Read the model definition and answer for the solid it produces. Units are mm, in the model's axes. Coordinates: 2 decimals unless noted, no trailing zeros. Loops run counter-clockwise (first coordinate to the right, second up) from the corner with the lowest first, then second, coordinate; pieces in that order, holes last.
Q1. Straight lines are drawn through the part: line 1 (Y direction, x = -27, z = 1.6); line 2 (X direction, y = 35.5, z = 1.4); line 3 (X direction, y = 50, z = 0.25). For each, find the intervals that lie inside material, in ascending order.
Q2. Section A-A (y = 59.5) is taken. Give the vertices of the cut face in (x, z).
Q3. Flat-ended cylindrical pins translate along their axes: P1, Ø2, axis at x = -15, y = 26.5, coming from the -Z side; P2, Ø0.6, axis at x = -27, z = 1.5, coming from the -Y side; P3, Ø0.6, axis at x = -35, z = 0.5, coming from the -Y side. Find the tip coordinate at first contact, or state that the pin passes through.
Q4. Section C-C (z = 0.65) is taken. Count the separate pieces of the cut face and the enclosed holes in it, then the cut area to 3 significant figures.
Q5. Section B-B (x = -42) is taken. Give the vertices of the cut face in (y, z), then the cut area to 3 significant figures.
from build123d import *

# Parameters (mm, degrees)
F0_R     = 1.6
F0_W     = 2
F0_H     = 3
F1_DEPTH = 2
F2_R     = 5
F3_R     = 2
F4_R     = 13.153232


with BuildPart() as f1:
    # F0 (on Top) → F1 (new body)
    with BuildSketch(Plane.XY):
        with Locations((-42.057751, 35.748998)):
            Circle(F0_R)
        with BuildLine():
            ThreePointArc((-13.157751, 35.748998), (-11.557751, 34.148998), (-9.957751, 35.748998))
            ThreePointArc((-9.957751, 35.748998), (-11.557751, 37.348998), (-13.157751, 35.748998))
        make_face()
        with Locations((-42.057751, 5.248998)):
            Circle(F0_R)
        with BuildLine():
            ThreePointArc((-13.157751, 5.248998), (-11.557751, 3.648998), (-9.957751, 5.248998))
            ThreePointArc((-9.957751, 5.248998), (-11.557751, 6.848998), (-13.157751, 5.248998))
        make_face()
        with BuildLine():
            ThreePointArc((-45.849798, 66.493904), (-45.855762, 66.371516), (-45.857751, 66.248998))
            Line((-45.857751, 66.248998), (-45.857751, 60.434222))
            Line((-45.857751, 60.434222), (-45.857751, 35.748998))
            Line((-45.857751, 35.748998), (-45.857751, 33.160256))
            Line((-45.857751, 33.160256), (-45.857751, 5.248998))
            Line((-45.857751, 5.248998), (-45.857751, -19.436226))
            Line((-45.857751, -19.436226), (-45.857751, -25.251002))
            Line((-45.857751, -25.251002), (-45.857751, -26.920806))
            ThreePointArc((-45.857751, -26.920806), (-40.539361, -28.348832), (-35.116938, -29.308968))
            ThreePointArc((-35.116938, -29.308968), (-26.575174, -26.898307), (-18.01507, -29.243015))
            ThreePointArc((-18.01507, -29.243015), (-12.838073, -28.295417), (-7.757751, -26.920806))
            Line((-7.757751, -26.920806), (-7.757751, -25.251002))
            Line((-7.757751, -25.251002), (-7.757751, -19.436226))
            Line((-7.757751, -19.436226), (-7.757751, 5.248998))
            Line((-7.757751, 5.248998), (-7.757751, 35.748998))
            Line((-7.757751, 35.748998), (-7.757751, 60.434222))
            Line((-7.757751, 60.434222), (-7.757751, 66.248998))
            ThreePointArc((-7.757751, 66.248998), (-7.759739, 66.371516), (-7.765703, 66.493904))
            ThreePointArc((-7.765703, 66.493904), (-11.655268, 70.022009), (-15.307751, 66.248998))
            ThreePointArc((-15.307751, 66.248998), (-26.807751, 65.147515), (-38.307751, 66.248998))
            ThreePointArc((-38.307751, 66.248998), (-41.960233, 70.022009), (-45.849798, 66.493904))
        make_face()
        with Locations((-42.057751, -23.592251)):
            Circle(F0_R, mode=Mode.SUBTRACT)
        with Locations((-35.116938, -24.283788)):
            Rectangle(F0_W, F0_H, mode=Mode.SUBTRACT)
        with Locations((-26.807751, -24.283788)):
            Rectangle(F0_W, F0_H, mode=Mode.SUBTRACT)
        with Locations((-42.057751, 5.248998)):
            Circle(F0_R, mode=Mode.SUBTRACT)
        with Locations((-18.498563, -24.283788)):
            Rectangle(F0_W, F0_H, mode=Mode.SUBTRACT)
        with Locations((-11.557751, -23.592251)):
            Circle(F0_R, mode=Mode.SUBTRACT)
        with BuildLine():
            ThreePointArc((-13.157751, 5.248998), (-11.557751, 6.848998), (-9.957751, 5.248998))
            ThreePointArc((-9.957751, 5.248998), (-11.557751, 3.648998), (-13.157751, 5.248998))
        make_face(mode=Mode.SUBTRACT)
        with Locations((-42.057751, 35.748998)):
            Circle(F0_R, mode=Mode.SUBTRACT)
        with Locations((-42.057751, 66.248998)):
            Circle(F0_R, mode=Mode.SUBTRACT)
        with BuildLine():
            ThreePointArc((-13.157751, 35.748998), (-11.557751, 37.348998), (-9.957751, 35.748998))
            ThreePointArc((-9.957751, 35.748998), (-11.557751, 34.148998), (-13.157751, 35.748998))
        make_face(mode=Mode.SUBTRACT)
        with BuildLine():
            ThreePointArc((-28.357751, 60.4842), (-26.807751, 62.0342), (-25.257751, 60.4842))
            Line((-25.257751, 60.4842), (-25.257751, 48.4842))
            ThreePointArc((-25.257751, 48.4842), (-26.807751, 46.9342), (-28.357751, 48.4842))
            Line((-28.357751, 48.4842), (-28.357751, 60.4842))
        make_face(mode=Mode.SUBTRACT)
        with Locations((-11.557751, 66.248998)):
            Circle(F0_R, mode=Mode.SUBTRACT)
    extrude(amount=F1_DEPTH)

    # F2
    f2_edges = [f1.edges().sort_by_distance(p)[0] for p in [
        (-35.116938, -29.308968, 1),
        (-18.01507, -29.243015, 1),
    ]]
    fillet(f2_edges, radius=F2_R)

    # F3
    f3_edges = [f1.edges().sort_by_distance(p)[0] for p in [
        (-7.757751, -26.920806, 1),
        (-45.857751, -26.920806, 1),
    ]]
    fillet(f3_edges, radius=F3_R)

    # F4
    f4_edges = [f1.edges().sort_by_distance(p)[0] for p in [
        (-38.307751, 66.248998, 1),
        (-15.307751, 66.248998, 1),
    ]]
    fillet(f4_edges, radius=F4_R)


solid = f1.part
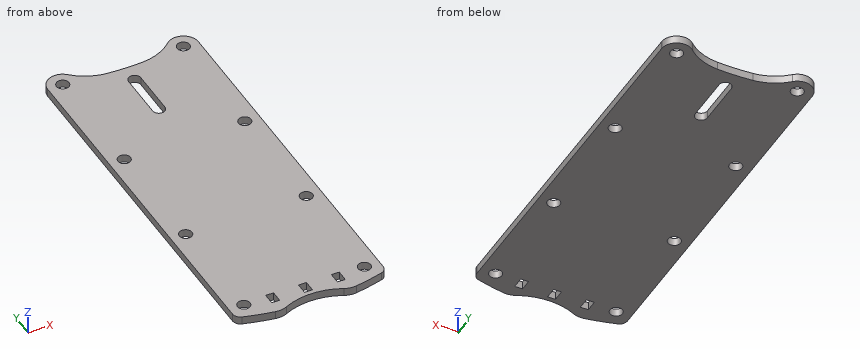
Numbers:
1. line 1: y = -26.91 to -25.78, -22.78 to 46.95, 62.02 to 65.15
1. line 2: x = -45.86 to -43.64, -40.48 to -13.14, -9.98 to -7.76
1. line 3: x = -45.86 to -28.36, -25.26 to -7.76
2. outline: (-45.86, 0) - (-28.36, 0) - (-28.36, 2) - (-45.86, 2) - close; (-25.26, 0) - (-7.76, 0) - (-7.76, 2) - (-25.26, 2) - close
3. P1: stops at z = 0
3. P2: stops at y = -26.92
3. P3: stops at y = -29.06
4. separate pieces: 1
4. enclosed holes: 12
4. area: 3,500 mm2
5. outline: (-28.01, 0) - (-25.19, 0) - (-25.19, 2) - (-28.01, 2) - close; (-21.99, 0) - (3.65, 0) - (3.65, 2) - (-21.99, 2) - close; (6.85, 0) - (34.15, 0) - (34.15, 2) - (6.85, 2) - close; (37.35, 0) - (64.65, 0) - (64.65, 2) - (37.35, 2) - close; (67.85, 0) - (70.02, 0) - (70.02, 2) - (67.85, 2) - close
5. area: 170 mm2
